from build123d import *

# Parameters (mm, degrees)
F1_DEPTH = 40


# Not quite as in the source:
# - the dataset's text gives a spline's control points without its knots; the knots are read off the source's solid


with BuildPart() as f1:
    # F0 (on Front) → F1 (new body)
    with BuildSketch(Plane.XZ):
        with BuildLine():
            Line((14.8645307095, 14.8645307095), (19.2446576564, 19.2446576564))
            ThreePointArc((19.2446576564, 19.2446576564), (10.4151336723, 25.1443569656), (0, 27.2160558609))
            Line((0, 27.2160558609), (0, 21.0216209277))
            ThreePointArc((0, 21.0216209277), (8.0446260505, 19.4214453153), (14.8645307095, 14.8645307095))
        make_face()
        with BuildLine():
            add(Edge.make_bspline(
                [(19.2446576564, 19.2446576564), (24.6689861063, 20.8169419681), (35.6038275727, 23.3831834597), (39.5588464284, 29.0400313178), (41.6940481575, 31.8752741371)],
                knots=[0, 0, 0, 0, 0.5609906845, 0.9958506588, 0.9958506588, 0.9958506588, 0.9958506588], degree=3))
            ThreePointArc((19.2446576564, 19.2446576564), (20.2037869779, 18.2351498041), (21.1100269664, 17.1779061036))
            add(Edge.make_bspline(
                [(21.1100269664, 17.1779061036), (21.932882048, 17.4106073742), (24.0175916845, 17.9893669374), (27.419341518, 18.9554948799), (30.5229232771, 19.9727275496), (32.8770808493, 20.9067554384), (34.2794910559, 21.5551214884), (35.3497904598, 22.1226810179), (36.1267174841, 22.5777216487), (36.8651895753, 23.0595386993), (37.7916316161, 23.7289766273), (38.8502830375, 24.6135981903), (40.3593073263, 26.1032349307), (41.3483421725, 27.3012382121), (41.9852374937, 28.1182048261), (42.0071509342, 28.1463677389)],
                knots=[0.0404952119, 0.0404952119, 0.0404952119, 0.0404952119, 0.125, 0.25, 0.375, 0.4375, 0.5, 0.53125, 0.5625, 0.59375, 0.625, 0.6875, 0.75, 0.875, 0.8794611677, 0.8794611677, 0.8794611677, 0.8794611677], degree=3))
            ThreePointArc((42.0071509342, 28.1463677389), (41.602326035, 29.9899743097), (41.6940481575, 31.8752741371))
        make_face()
        with BuildLine():
            ThreePointArc((21.1100269664, 17.1779061036), (20.2037869779, 18.2351498041), (19.2446576564, 19.2446576564))
            Line((19.2446576564, 19.2446576564), (14.8645307095, 14.8645307095))
            ThreePointArc((14.8645307095, 14.8645307095), (19.4214453153, 8.0446260505), (21.0216209277, 0))
            Line((21.0216209277, 0), (27.2160558609, 0))
            ThreePointArc((27.2160558609, 0), (27.1163610427, 2.3273720003), (26.8180069698, 4.6376932618))
            ThreePointArc((26.8180069698, 4.6376932618), (24.7707154474, 11.2749879312), (21.1100269664, 17.1779061036))
        make_face()
        with BuildLine():
            Line((0, 21.0216209277), (0, 27.2160558609))
            ThreePointArc((0, 27.2160558609), (-19.2446576564, -19.2446576564), (27.2160558609, 0))
            Line((27.2160558609, 0), (21.0216209277, 0))
            ThreePointArc((21.0216209277, 0), (-14.8645307095, -14.8645307095), (0, 21.0216209277))
        make_face()
        with BuildLine():
            ThreePointArc((55.8771080393, 30.5882225912), (49.3733508957, 37.7088912623), (41.6940481575, 31.8752741371))
            ThreePointArc((41.6940481575, 31.8752741371), (41.602326035, 29.9899743097), (42.0071509342, 28.1463677389))
            ThreePointArc((42.0071509342, 28.1463677389), (42.8595475903, 26.5025969086), (44.1054687849, 25.1328367183))
            ThreePointArc((44.1054687849, 25.1328367183), (45.2874793483, 24.3200561007), (46.60794615, 23.7595842193))
            ThreePointArc((46.60794615, 23.7595842193), (52.9679994545, 24.8317552686), (55.8771080393, 30.5882225912))
        make_face()
        with BuildLine():
            ThreePointArc((53.7271809085, 30.5882225912), (48.8098673687, 25.588906343), (43.7299157288, 30.4228722856))
            ThreePointArc((43.7299157288, 30.4228722856), (48.6444944483, 35.5875388394), (53.7271809085, 30.5882225912))
        make_face(mode=Mode.SUBTRACT)
        with BuildLine():
            ThreePointArc((26.8180069698, 4.6376932618), (27.1163610427, 2.3273720003), (27.2160558609, 0))
            add(Edge.make_bspline(
                [(27.2160558609, 0), (30.4118613071, 6.1535153267), (36.1085642411, 17.1225033402), (43.4048284049, 21.734764605), (46.60794615, 23.7595842193)],
                knots=[0, 0, 0, 0, 0.5609920336, 1, 1, 1, 1], degree=3))
            ThreePointArc((46.60794615, 23.7595842193), (45.2874793483, 24.3200561007), (44.1054687849, 25.1328367183))
            add(Edge.make_bspline(
                [(26.8180069698, 4.6376932618), (26.9287178391, 4.8472219351), (27.763643844, 6.4224538826), (29.3467248011, 9.3274546207), (31.2690824478, 12.5225076847), (32.8847011617, 14.9107917128), (33.9343354718, 16.3212905579), (34.8023613487, 17.3919432452), (35.693376161, 18.4237208714), (36.8375292868, 19.6172523124), (38.236939936, 20.9022131544), (40.1258580525, 22.4490696098), (42.0976326485, 23.8377548069), (43.5711967417, 24.7916786126), (44.1054687849, 25.1328367183)],
                knots=[0.1058501262, 0.1058501262, 0.1058501262, 0.1058501262, 0.125, 0.25, 0.375, 0.4375, 0.5, 0.53125, 0.5625, 0.625, 0.6875, 0.75, 0.875, 0.9471213486, 0.9471213486, 0.9471213486, 0.9471213486], degree=3))
        make_face()
    extrude(amount=F1_DEPTH)


solid = f1.part
Geometry: final body of the model. Coordinates: model frame, mm. Give positions to 0.01 mm unless a question says otherwise; leave off trailing zeros. Loops run counter-clockwise (first coordinate to the right, second up) from the corner with the lowest first, then second, coordinate; pieces in that order, holes last. Notation, with made-up numbers: (11, 39) -> (70, 39) arc R14 ccw to (70, 57) -> close; hole circle Ø1 at (79.25, -11). An arc over 180 degrees is marked (long way). Put each result on its own line as item: value.
1. Pin query (flat end, axial travel): P1, Ø12, axis at x = 3, y = -22, coming from the -Z side; P2, Ø1, axis at y = -25, z = 13.5, coming from the -X side; P3, Ø5, axis at y = -21.5, z = -10, coming from the -X side; P4, Ø6, axis at x = -1, y = -27, coming from the +Z side. Return the tip coordinate at first contact, or that it passes through.
Taken from the geometry:
P1: stops at z = -27.22
P2: stops at x = -23.91
P3: stops at x = -26.16
P4: stops at z = 27.22
2. Ray query, line 1 along X through (y, z) = (-26, 0); line 2 along X through (y, z) = (-26, 11); line 3 along X through (y, z) = (-20.5, -12.5). Return the intervals inside material, ascending. Write a range as [from, to].
Taken from the geometry:
line 1: x = [-27.22, -21.02], [21.02, 27.22]
line 2: x = [-24.89, -17.91], [17.91, 24.89], [30.36, 33.3]
line 3: x = [-24.18, -16.9], [16.9, 24.18]
3. Pull-direction query (X, two-part tool) for faces 1 (the flat face through (17, 0, 13)), 2 (the cylindrical face through (42.845, -19.72, 26.524)); classes: released by +X, released by -X, zero draft, split by the parting line, or undercut.
Taken from the geometry:
face 1: zero draft
face 2: undercut
4. Cut plane A-A (z = -18.5). Return the cut outline in (x, y).
Taken from the geometry:
outline: (-19.96, -40) -> (-9.98, -40) -> (-9.98, 0) -> (-19.96, 0) -> close; (9.98, -40) -> (19.96, -40) -> (19.96, 0) -> (9.98, 0) -> close
5. Cut plane B-B (x = -8.5). Return the cut outline in (y, z).
Taken from the geometry:
outline: (-40, -25.85) -> (0, -25.85) -> (0, -19.23) -> (-40, -19.23) -> close; (-40, 19.23) -> (0, 19.23) -> (0, 25.85) -> (-40, 25.85) -> close
6. Cut plane C-C (y = -9.5). Count the separate pieces of the cut face and the enclosed holes in it, plus the area to 3 significant figures.
Taken from the geometry:
separate pieces: 1
enclosed holes: 3
area: 1,160 mm2
